Read the model definition and answer for the solid it produces. Units are mm, in the model's axes. Coordinates: 2 decimals unless noted, no trailing zeros. Write each loop counter-clockwise with the first axis right and the second up, starting at its lowest first coordinate (ties: lowest second). Pieces come first, ordered by that corner, then holes. Notation, with made-up numbers: M 73,1 L 113,1 A14 cw 113,26 Z; hole C 31,20.5 d1. An arc over 180 degrees is marked long. Write item = value, one per line.
from build123d import *

# Parameters (mm, degrees)
F0_W     = 439.997
F0_H     = 270.002
F1_DEPTH = 4
F2_T     = -3
F4_SIZE  = 1.778
F3_W     = 5
F3_H     = 5
F5_DEPTH = 1
F6_R     = 2.5
F7_DEPTH = 4.001
F8_R     = 4
F9_DEPTH = 4.001


with BuildPart() as f1:
    # F0 (on Front) → F1 (new body)
    with BuildSketch(Plane.XZ):
        with Locations((-2.7703095811, 18.9870057008)):
            Rectangle(F0_W, F0_H)
    extrude(amount=F1_DEPTH)

    # F2
    f2_openings = [f1.faces().sort_by_distance(p)[0] for p in [
        (-2.77031, 0, 18.987006),
    ]]
    offset(amount=F2_T, openings=f2_openings)

    # F4
    f4_edges = [f1.edges().sort_by_distance(p)[0] for p in [
        (-222.76881, -2, -116.013994),
        (-222.76881, -2, 153.988006),
        (217.22819, -2, 153.988006),
        (217.22819, -2, -116.013994),
    ]]
    chamfer(f4_edges, length=F4_SIZE)

    # F3 (on face) → F5 (join, through all)
    with BuildSketch(Plane(origin=(0, -1, 0), x_dir=(-1, 0, 0), z_dir=(0, 1, 0))):
        with Locations((217.2688095811, -110.5139942992)):
            Rectangle(F3_W, F3_H)
        with Locations((217.2688095811, 148.4880057008)):
            Rectangle(F3_W, F3_H)
        with Locations((-211.7281904189, -110.5139942992)):
            Rectangle(F3_W, F3_H)
    extrude(amount=F5_DEPTH)

    # F6 (on face) → F7 (cut, through all)
    with BuildSketch(Plane.XZ.offset(4)):
        with Locations((-182.7688095811, -58.0139942992)):
            Circle(F6_R)
        with Locations((-188.3311154799, -58.8949770059)):
            Circle(F6_R)
        with Locations((-193.3489441224, -61.4516884005)):
            Circle(F6_R)
        with Locations((-197.3311154799, -65.433859758)):
            Circle(F6_R)
        with Locations((-199.8878268745, -70.4516884005)):
            Circle(F6_R)
        with Locations((-200.7688095811, -76.0139942992)):
            Circle(F6_R)
        with Locations((-199.8878268745, -81.576300198)):
            Circle(F6_R)
        with Locations((-197.3311154799, -86.5941288405)):
            Circle(F6_R)
        with Locations((-193.3489441224, -90.576300198)):
            Circle(F6_R)
        with Locations((-188.3311154799, -93.1330115926)):
            Circle(F6_R)
        with Locations((-182.7688095811, -94.0139942992)):
            Circle(F6_R)
        with Locations((-177.2065036824, -93.1330115926)):
            Circle(F6_R)
        with Locations((-172.1886750399, -90.576300198)):
            Circle(F6_R)
        with Locations((-168.2065036824, -86.5941288405)):
            Circle(F6_R)
        with Locations((-182.7688095811, -64.0139942992)):
            Circle(F6_R)
        with Locations((-187.9754144506, -65.2023678844)):
            Circle(F6_R)
        with Locations((-192.1507873708, -68.5321166769)):
            Circle(F6_R)
        with Locations((-194.4679445273, -73.3437430918)):
            Circle(F6_R)
        with Locations((-194.4679445273, -78.6842455067)):
            Circle(F6_R)
        with Locations((-192.1507873708, -83.4958719215)):
            Circle(F6_R)
        with Locations((-187.9754144506, -86.8256207141)):
            Circle(F6_R)
        with Locations((-182.7688095811, -88.0139942992)):
            Circle(F6_R)
        with Locations((-177.5622047117, -86.8256207141)):
            Circle(F6_R)
        with Locations((-173.3868317915, -83.4958719215)):
            Circle(F6_R)
        with Locations((-182.7688095811, -70.0139942992)):
            Circle(F6_R)
        with Locations((-187.459798476, -72.2730554881)):
            Circle(F6_R)
        with Locations((-188.6183770542, -77.349119903)):
            Circle(F6_R)
        with Locations((-185.3721120159, -81.4198075067)):
            Circle(F6_R)
        with Locations((-180.1655071464, -81.4198075067)):
            Circle(F6_R)
        with Locations((-176.9192421081, -77.349119903)):
            Circle(F6_R)
        with Locations((-178.0778206863, -72.2730554881)):
            Circle(F6_R)
        with Locations((-182.7688095811, -76.0139942992)):
            Circle(F6_R)
        with Locations((-165.6497922878, -81.576300198)):
            Circle(F6_R)
        with Locations((-164.7688095811, -76.0139942992)):
            Circle(F6_R)
        with Locations((-165.6497922878, -70.4516884005)):
            Circle(F6_R)
        with Locations((-171.069674635, -78.6842455067)):
            Circle(F6_R)
        with Locations((-171.069674635, -73.3437430918)):
            Circle(F6_R)
        with Locations((-168.2065036824, -65.433859758)):
            Circle(F6_R)
        with Locations((-172.1886750399, -61.4516884005)):
            Circle(F6_R)
        with Locations((-177.2065036824, -58.8949770059)):
            Circle(F6_R)
        with Locations((-173.3868317915, -68.5321166769)):
            Circle(F6_R)
        with Locations((-177.5622047117, -65.2023678844)):
            Circle(F6_R)
    extrude(amount=-F7_DEPTH, mode=Mode.SUBTRACT)

    # F8 (on face) → F9 (cut, through all)
    with BuildSketch(Plane.XZ.offset(4)):
        with Locations((137.2281904189, 113.9880057008)):
            Circle(F8_R)
        with Locations((127.9576805876, 112.5197011896)):
            Circle(F8_R)
        with Locations((119.5946328501, 108.258515532)):
            Circle(F8_R)
        with Locations((112.9576805876, 101.6215632695)):
            Circle(F8_R)
        with Locations((108.69649493, 93.258515532)):
            Circle(F8_R)
        with Locations((107.2281904189, 83.9880057008)):
            Circle(F8_R)
        with Locations((108.69649493, 74.7174958695)):
            Circle(F8_R)
        with Locations((112.9576805876, 66.354448132)):
            Circle(F8_R)
        with Locations((119.5946328501, 59.7174958695)):
            Circle(F8_R)
        with Locations((127.9576805876, 55.4563102119)):
            Circle(F8_R)
        with Locations((137.2281904189, 53.9880057008)):
            Circle(F8_R)
        with Locations((146.4987002501, 55.4563102119)):
            Circle(F8_R)
        with Locations((154.8617479876, 59.7174958695)):
            Circle(F8_R)
        with Locations((161.4987002501, 66.354448132)):
            Circle(F8_R)
        with Locations((137.2281904189, 103.9880057008)):
            Circle(F8_R)
        with Locations((128.5505156365, 102.0073830588)):
            Circle(F8_R)
        with Locations((121.5915607695, 96.4578017379)):
            Circle(F8_R)
        with Locations((117.7296321752, 88.4384243799)):
            Circle(F8_R)
        with Locations((117.7296321752, 79.5375870216)):
            Circle(F8_R)
        with Locations((121.5915607695, 71.5182096636)):
            Circle(F8_R)
        with Locations((128.5505156365, 65.9686283427)):
            Circle(F8_R)
        with Locations((137.2281904189, 63.9880057008)):
            Circle(F8_R)
        with Locations((145.9058652012, 65.9686283427)):
            Circle(F8_R)
        with Locations((152.8648200682, 71.5182096636)):
            Circle(F8_R)
        with Locations((137.2281904189, 93.9880057008)):
            Circle(F8_R)
        with Locations((129.4098755942, 90.2229037193)):
            Circle(F8_R)
        with Locations((127.478911297, 81.7627963612)):
            Circle(F8_R)
        with Locations((132.8893530277, 74.9783170217)):
            Circle(F8_R)
        with Locations((141.56702781, 74.9783170217)):
            Circle(F8_R)
        with Locations((146.9774695407, 81.7627963612)):
            Circle(F8_R)
        with Locations((145.0465052435, 90.2229037193)):
            Circle(F8_R)
        with Locations((137.2281904189, 83.9880057008)):
            Circle(F8_R)
        with Locations((165.7598859077, 74.7174958695)):
            Circle(F8_R)
        with Locations((167.2281904189, 83.9880057008)):
            Circle(F8_R)
        with Locations((165.7598859077, 93.258515532)):
            Circle(F8_R)
        with Locations((156.7267486625, 79.5375870216)):
            Circle(F8_R)
        with Locations((156.7267486625, 88.4384243799)):
            Circle(F8_R)
        with Locations((161.4987002501, 101.6215632695)):
            Circle(F8_R)
        with Locations((154.8617479876, 108.258515532)):
            Circle(F8_R)
        with Locations((146.4987002501, 112.5197011896)):
            Circle(F8_R)
        with Locations((152.8648200682, 96.4578017379)):
            Circle(F8_R)
        with Locations((145.9058652012, 102.0073830588)):
            Circle(F8_R)
    extrude(amount=-F9_DEPTH, mode=Mode.SUBTRACT)


solid = f1.part
Item 1: For a pull along X with two mould halves and no side action, classify faces 1 (the face through (-6, -4, 21)), 2 (the face through (131.653, -2.521, 110.988)) as released by +X, released by -X, zero draft, split by the parting line, or undercut.
Worked answers:
face_1 = zero draft
face_2 = undercut
Item 2: Find section A-A (z = 12.5). Determine the outline of the cut face in (x, y).
Worked answers:
outline = M -222.77,-4 L 217.23,-4 L 217.23,0 L 214.23,0 L 214.23,-1 L -219.77,-1 L -219.77,0 L -222.77,0 Z
Item 3: Find section B-B (x = 13). Determine the outline of the cut face in (y, z), and give its area (3 significant figures).
Worked answers:
outline = M -4,-116.01 L 0,-116.01 L 0,-113.01 L -1,-113.01 L -1,150.99 L 0,150.99 L 0,153.99 L -4,153.99 Z
area = 816 mm²
Item 4: Consider line 1 along Z through (x, y) = (-151, -0.4); line 2 along X through (y, z) = (-0.9, 115.5); line 3 along X through (y, z) = (-3.8, 66.5). Determine where each line is inside the solid, lowest interval first. Write a range as from..to.
Worked answers:
line_1 = -116.01..-113.01, 150.99..153.99
line_2 = -222.77..-219.77, 214.23..217.23
line_3 = -222.77..108.96, 116.96..124.59, 132.52..134.12, 140.34..141.94, 149.87..157.5, 165.5..217.23
Item 5: Find section C-C (y = -2.3). State how many separate pieces and enclosed holes the cut face has, and give its area (3 significant figures).
Worked answers:
separate_pieces = 1
enclosed_holes = 84
area = 116,000 mm²
Item 6: A flat-ended cylindrical pin translates along its axis: pin 1 (5 mm diameter, centred on x = 112.5, z = -61.5, fed in from +Y). Find the tip coordinate at first contact, or state that the pin passes through.
Worked answers:
pin_1 = -1
